Geometry check sheet. Reference: the model listing, model coordinates, mm. Face numbers are marked on the shaded views. A direction names the side the tool comes from. Round coordinates to 2 decimals unless told otherwise and drop trailing zeros. Loops run counter-clockwise (first coordinate to the right, second up) from the corner with the lowest first, then second, coordinate; pieces in that order, holes last. Notation, with made-up numbers: (23.25, 34.5) - (40.25, 34.5) arc R22 cw to (40.25, 58.5) - close; hole circle Ø2 at (19, 56). An arc over 180 degrees is marked (long way). Answer in a Markdown table with one row per item. Add a question column.
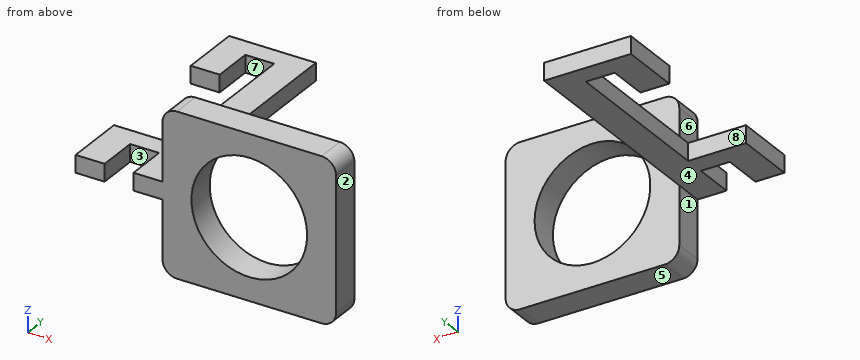
Autodesk Inventor part; units mm, degrees
ref_plane "YZ Plane" through (0, 0, 0) normal (1, 0, 0) x (0, 1, 0)
ref_plane "XZ Plane" through (0, 0, 0) normal (0, 1, 0) x (-1, 0, 0)
ref_plane "XY Plane" through (0, 0, 0) normal (0, 0, 1) x (1, 0, 0)
sketch "Sketch1" plane through (0, 0, 0) normal (0, 0, 1) x (1, 0, 0)
  line L0 (0, 6.35) -> (0, 53.34)
  line L1 (0, 53.34) -> (-19.05, 53.34)
  line L2 (-19.05, 53.34) -> (-19.05, 55.245)
  line L3 (-12.7, 48.895) -> (-6.35, 48.895)
  line L4 (-6.35, 48.895) -> (-6.35, 13.335)
  line L5 (-6.35, 13.335) -> (-19.05, 13.335)
  line L6 (-19.05, 13.335) -> (-19.05, 12.7)
  line L7 (-12.7, 8.89) -> (-6.35, 8.89)
  line L8 (-6.35, 8.89) -> (-6.35, 0)
  line L9 (-6.35, 0) -> (0, 0)
  line L10 (-19.05, 55.245) -> (-19.05, 40.005)
  line L11 (-19.05, 40.005) -> (-12.7, 40.005)
  line L12 (-12.7, 40.005) -> (-12.7, 48.895)
  line L13 (-19.05, 12.7) -> (-19.05, 0)
  line L14 (-19.05, 0) -> (-12.7, 0)
  line L15 (-12.7, 0) -> (-12.7, 8.89)
  line L16 (0, 0) -> (0, 6.35)
  point P0 (-19.05, 53.34)
  point P1 (-19.05, 11.43)
  dimension "d1" = 35.56
  dimension "d2" = 4.445
  dimension "d3" = 4.445
  dimension "d4" = 6.35
  dimension "d6" = 6.35
  dimension "d7" = 6.35
  dimension "d13" = 13.335
  dimension "d14" = 13.335
extrude "Extrusion1" add sketch "Sketch1" along normal mid plane 3.81
sketch "Sketch2" plane through (0, 0, 0) normal (0, 0, 1) x (1, 0, 0)
  line L0 (0, 53.34) -> (0, 0)
  line L1 (0, 0) -> (38.1, 0)
  line L2 (38.1, 0) -> (38.1, 6.35)
  line L3 (38.1, 6.35) -> (0, 6.35)
  dimension "d15" = 38.1
  dimension "d16" = 6.35
extrude "Extrusion2" add sketch "Sketch2" along normal mid plane 35.56
sketch "Sketch3" plane through (0, 6.35, 17.78) normal (0, 1, 0) x (1, 0, 0)
  circle A0 centre (19.05, 17.78) radius 12.7
  point P0 (0, 17.78)
  dimension "d19" = 25.4
extrude "Extrusion3" cut sketch "Sketch3" against normal through all
fillet "Fillet1" radius 3.175 4 edges at (38.1, 3.175, 17.78) (38.1, 3.175, -17.78) (0, 3.175, -17.78) (0, 3.175, 17.78)
equation "\"d11\" = width"
equation "\"width\" = 3.81"
properties part number "round_1_0_inchHoleV01"
Q1. Scan lines: line 1 (Z direction, x = 19.05, y = 2); line 2 (X direction, y = 1.75, z = 0); line 3 (Y direction, x = -9.5, z = 0.5) (3 decimals). Record each from-to range of solid material in increasing order. Write a range as from..to.
Q2. Cross-section at B-B, the plane x = 19.05. Enter the section's corners in (y, z), plus the area to 3 significant figures.
Q3. Release check for a two-part mould opening along X. For the marked faces 1, 2 and 3 record: +X half, -X half, draft (parallel to the pull), parting line (faces both ways), or undercut.
Q4. Cross-section at C-C, the plane z = 0. Enter the section's corners in (x, y) (3 decimals).
Q5. Depth check by flat-ended pin: P1, Ø3, axis at y = 23.5, z = 0, coming from the +X side; P2, Ø3, axis at x = -8.5, z = -0.5, coming from the -Y side; P3, Ø2, axis at x = -4.5, y = 18, coming from the +Z side (3 decimals); P4, Ø4, axis at x = -15, z = 0.5, coming from the -Y side. Enter the tip coordinate at first touch or a pass-through.
Q6. Cross-section at A-A, the plane y = 43.5. Enter the section's corners in (x, z) (3 decimals), plus the area to 3 significant figures.
Q7. Set-up check for the marked faces 4, 5, 6, 7 and 8: record each of +Z, -Z, +X, -X, +Y, -Y from which the full face is reachable in a straight line by a thin tool's end or side.
Q8. Cross-section at D-D, the plane y = 31.5. Enter the section's corners in (x, z) (3 decimals), plus the area to 3 significant figures.
Check sheet entries:
| question | item | result |
|---|---|---|
| 1 | line 1 | -17.78..-12.7, 12.7..17.78 |
| 1 | line 2 | -19.05..-12.7, -6.35..6.35, 31.75..38.1 |
| 1 | line 3 | 8.89..13.335, 48.895..53.34 |
| 2 | outline | (0, -17.78) - (6.35, -17.78) - (6.35, -12.7) - (0, -12.7) - close; (0, 12.7) - (6.35, 12.7) - (6.35, 17.78) - (0, 17.78) - close |
| 2 | area | 64.5 mm² |
| 3 | face 1 | -X half |
| 3 | face 2 | +X half |
| 3 | face 3 | undercut |
| 4 | outline | (-19.05, 0) - (-12.7, 0) - (-12.7, 8.89) - (-6.35, 8.89) - (-6.35, 0) - (6.35, 0) - (6.35, 6.35) - (0, 6.35) - (0, 53.34) - (-19.05, 53.34) - (-19.05, 40.005) - (-12.7, 40.005) - (-12.7, 48.895) - (-6.35, 48.895) - (-6.35, 13.335) - (-19.05, 13.335) - close; (31.75, 0) - (38.1, 0) - (38.1, 6.35) - (31.75, 6.35) - close |
| 5 | P1 | x = 0 |
| 5 | P2 | y = 8.89 |
| 5 | P3 | z = 1.905 |
| 5 | P4 | y = 0 |
| 6 | outline | (-19.05, -1.905) - (-12.7, -1.905) - (-12.7, 1.905) - (-19.05, 1.905) - close; (-6.35, -1.905) - (0, -1.905) - (0, 1.905) - (-6.35, 1.905) - close |
| 6 | area | 48.4 mm² |
| 7 | face 4 | -Z, -X, +Y, -Y |
| 7 | face 5 | -Z, +X, -X, +Y, -Y |
| 7 | face 6 | +Z, -X, +Y, -Y |
| 7 | face 7 | +Z, -Z |
| 7 | face 8 | +Z, -Z, -X |
| 8 | outline | (-6.35, -1.905) - (0, -1.905) - (0, 1.905) - (-6.35, 1.905) - close |
| 8 | area | 24.2 mm² |
